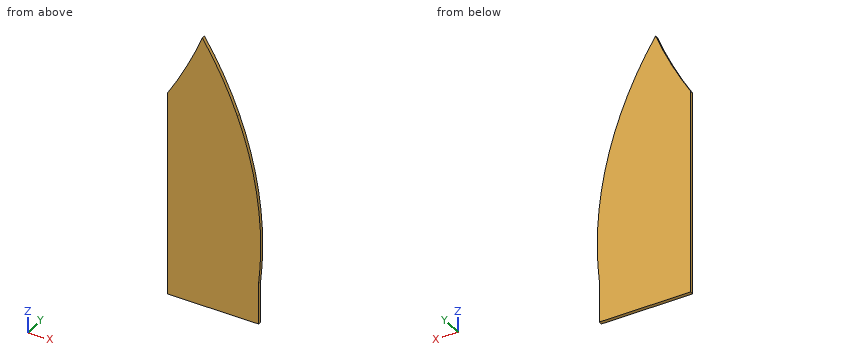
```python
from build123d import *

# Parameters (mm, degrees)
F0_W     = 25.4
F0_H     = 203.2
F0_H_2   = 101.6
F0_W_2   = 63.5
F0_W_3   = 38.1
F1_DEPTH = 6.35


with BuildPart() as f1:
    # F0 (on Front) → F1 (new body)
    with BuildSketch(Plane.XZ):
        with Locations((12.7, 101.6)):
            Rectangle(F0_W, F0_H)
        with Locations((12.7, 254)):
            Rectangle(F0_W, F0_H_2)
        with BuildLine():
            ThreePointArc((25.4, 349.25), (13.0471808847, 326.826610923), (0, 304.8))
            Line((0, 304.8), (25.4, 304.8))
            Line((25.4, 304.8), (25.4, 349.25))
        make_face()
        with BuildLine():
            Line((25.4, 349.25), (25.4, 304.8))
            Line((25.4, 304.8), (63.5, 304.8))
            Line((63.5, 304.8), (63.5, 431.8))
            ThreePointArc((63.5, 431.8), (45.5956444739, 389.996241012), (25.4, 349.25))
        make_face()
        with BuildLine():
            Line((63.5, 431.8), (63.5, 304.8))
            Line((63.5, 304.8), (127, 304.8))
            ThreePointArc((127, 304.8), (98.6420785739, 369.996039287), (63.5, 431.8))
        make_face()
        with Locations((95.25, 254)):
            Rectangle(F0_W_2, F0_H_2)
        with Locations((44.45, 254)):
            Rectangle(F0_W_3, F0_H_2)
        Polygon((25.4, 203.2), (25.4, 0), (50.8, 0), (63.5, 0), (63.5, 203.2), align=None)
        with Locations((95.25, 101.6)):
            Rectangle(F0_W_2, F0_H)
        Polygon((152.4, 203.2), (127, 203.2), (127, 0), (130.463650802, 0), (152.4, 0), align=None)
        with BuildLine():
            Line((152.4, 0), (165.1, 0))
            ThreePointArc((165.1, 0), (168.0222390688, 35.93060895), (168.9972698039, 71.9666666667))
            ThreePointArc((168.9972698039, 71.9666666667), (158.4139149447, 190.2619875611), (127, 304.8))
            Line((127, 304.8), (127, 203.2))
            Line((127, 203.2), (152.4, 203.2))
            Line((152.4, 203.2), (152.4, 0))
        make_face()
        with BuildLine():
            Line((25.4, 0), (0, 0))
            Line((0, 0), (0, -76.2))
            Line((0, -76.2), (152.3172585759, -76.2))
            ThreePointArc((152.3172585759, -76.2), (159.8138971323, -38.2854114575), (165.1, 0))
            Line((165.1, 0), (152.4, 0))
            Line((152.4, 0), (130.463650802, 0))
            Line((130.463650802, 0), (127, 0))
            Line((127, 0), (63.5, 0))
            Line((63.5, 0), (50.8, 0))
            Line((50.8, 0), (25.4, 0))
        make_face()
        with BuildLine():
            ThreePointArc((165.1, 0), (159.8138971323, -38.2854114575), (152.3172585759, -76.2))
            Line((152.3172585759, -76.2), (165.1, -76.2))
            Line((165.1, -76.2), (165.1, 0))
        make_face()
    extrude(amount=F1_DEPTH)


solid = f1.part
```
Model file for the job. Use its own axes, mm. Give positions to 0.01 mm unless a question says otherwise; leave off trailing zeros. Loops run counter-clockwise (first coordinate to the right, second up) from the corner with the lowest first, then second, coordinate; pieces in that order, holes last. Notation, with made-up numbers: (12, 69) -> (31, 69) arc R13 cw to (31, 76) -> close; hole circle Ø3 at (-27, -22.5). An arc over 180 degrees is marked (long way). Use CSV: the item, a comma, the result in double quotes. Start each with the question number.
1) Flat gauge pin, fed straight in: pin 1 Ø3 at (y, z) = (-2, -43.5) entering from +X. Where does the tip first touch, or does it go through?
2) Slice it at A-A on y = -1.75. Give the cut face in (x, z) (1 decimal), plus the area to 3 significant figures.
3) Slice it at B-B on z = -15.5. Give the cut face in (x, y).
4) Slice it at C-C on x = 70. Give the cut face in (y, z).
5) Wall check: line 1 (X direction, y = -2.5, z = -41); line 2 (X direction, y = -2.25, z = 261); line 3 (Z direction, x = 116, y = -1.5). Give the ranges that are in metal, low to high.
Computed values:
1,pin 1,"stops at x = 165.1"
2,outline,"(0, -76.2) -> (165.1, -76.2) -> (165.1, 0) arc R666.4 ccw to (63.5, 431.8) arc R819.5 cw to (0, 304.8) -> close"
2,area,"68,900 mm^2"
3,outline,"(0, -6.35) -> (165.1, -6.35) -> (165.1, 0) -> (0, 0) -> close"
4,outline,"(-6.35, -76.2) -> (0, -76.2) -> (0, 421.46) -> (-6.35, 421.46) -> close"
5,line 1,"x = 0 to 165.1"
5,line 2,"x = 0 to 141.62"
5,line 3,"z = -76.2 to 332.4"
